CAD build for the part. Positions are in the model's coordinates, mm. Face numbers are marked on the shaded views. Give positions to 0.01 mm unless a question says otherwise; leave off trailing zeros. Write each loop counter-clockwise with the first axis right and the second up, starting at its lowest first coordinate (ties: lowest second). Pieces come first, ordered by that corner, then holes. Notation, with made-up numbers: M 7.5,39 L 23.5,39 A19 cw 23.5,67 Z; hole C 33.5,-11.5 d2. An arc over 180 degrees is marked long. One line per question, with ' | ' between items. Start each with the question number.
1. Cut at A-A, the plane x = 8. Write the cut outline in (y, z).
2. Flat gauge pins, fed straight in: pin 1 (4 mm diameter, centred on y = -16, z = 90.5, fed in from +X); pin 2 (2 mm diameter, centred on x = 13.5, y = -12.5, fed in from +Z); pin 3 (3 mm diameter, centred on x = 6.5, z = 79, fed in from -Y). Where does each tip first touch, or does it go through?
3. Pull direction Y, two halves, no side cores. Call the marked faces 1, 2 and 3: released by +Y, released by -Y, zero draft, split by the parting line, or undercut.
4. Wall check: L1, parallel to Z at x = 5, y = -8; L2, parallel to Y at x = 7, z = 73; L3, parallel to X at y = -6.5, z = 76. Give the ranges that are in metal, low to high.
5. Cut at C-C, the plane z = 90. Write the cut outline in (x, y), then the cut area to 3 significant figures.
6. Cut at B-B, the plane z = 66. Write the cut outline in (x, y), then the cut area to 3 significant figures.
7. Cut at D-D, the plane z = 73. Write the cut outline in (x, y), then the cut area to 3 significant figures.
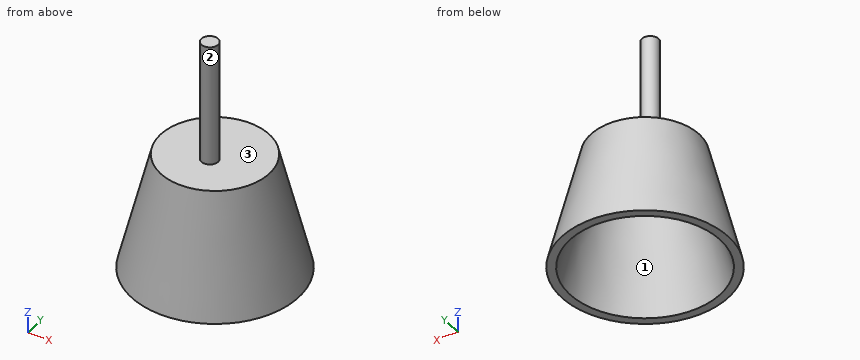
```python
from build123d import *

# Parameters (mm, degrees)
CYLINDER086_R     = 2
CYLINDER086_DEPTH = 30


with BuildPart() as cylindre082:
    # Cylinder086 → Cylinder086 (new body)
    with BuildSketch(Plane(origin=(8, -13, 88), x_dir=(1, 0, 0), z_dir=(0, 0, 1))):
        Circle(CYLINDER086_R)
    extrude(amount=CYLINDER086_DEPTH)


with BuildPart() as obj1:
    # Cone017 → Cone017 (revolve)
    with BuildSketch(Plane(origin=(8, -11, 73), x_dir=(-1, 0, 0), z_dir=(0, 1, 0))):
        Polygon((0, 0), (18, 0), (11, 26), (0, 26), align=None)
    revolve(axis=Axis((8, -11, 73), (0, 0, 1)))


with BuildPart() as fusion047:
    # Cone018 → Cone018 (revolve)
    with BuildSketch(Plane(origin=(8, -11, 73), x_dir=(-1, 0, 0), z_dir=(0, 1, 0))):
        Polygon((0, 0), (20, 0), (13, 28), (0, 28), align=None)
    revolve(axis=Axis((8, -11, 73), (0, 0, 1)))

    # Cut044: cut obj1
    add(obj1.part, mode=Mode.SUBTRACT)


with BuildPart() as fusion047_1:
    # Cut044 placement: moved
    add(fusion047.part.moved(Location((0, 0, -12))))

    # Fusion047: union Cylindre082
    add(cylindre082.part)


solid = fusion047_1.part
```
Here are the results:
1) outline: M -31,61 L -29,61 L -22,87 L 0,87 L 7,61 L 9,61 L 2,89 L -11,89 L -11,118 L -15,118 L -15,89 L -24,89 Z
2) pin 1: x = 20.47 | pin 2: z = 89 | pin 3: y = -26.82
3) face 1: undercut | face 2: split by the parting line | face 3: zero draft
4) L1: 87 to 89 | L2: -27.97 to -25.74, 3.74 to 5.97 | L3: -7.61 to -5.22, 21.22 to 23.61
5) outline: C 8,-13 d4 | area: 12.6 mm^2
6) outline: C 8,-11 d37.5; hole C 8,-11 d33.31 | area: 233 mm^2
7) outline: C 8,-11 d34; hole C 8,-11 d29.54 | area: 223 mm^2
